Read the model definition and answer for the solid it produces. Units are mm, in the model's axes. Face numbers are marked on the shaded views. A direction names the side the tool comes from. Give positions to 0.01 mm unless a question says otherwise; leave off trailing zeros. Order: outer loops, then holes, each group sorted by start corner. A loop starts at its lowest first (then second) coordinate and runs counter-clockwise, first axis right, second up.
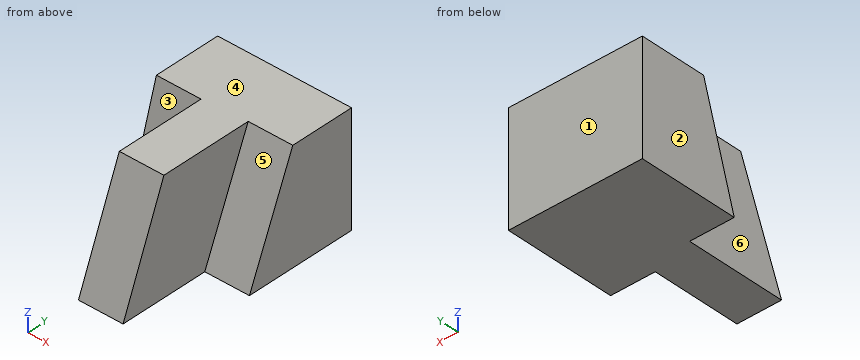
```python
from build123d import *

# Parameters (mm, degrees)
F0_W     = 38.1
F0_H     = 31.75
F1_DEPTH = 57.15
F3_DEPTH = 12.7
F5_DEPTH = 12.7
F7_DEPTH = 25.4


with BuildPart() as f1:
    # F0 (on Front) → F1 (new body)
    with BuildSketch(Plane.XZ):
        with Locations((19.05, 15.875)):
            Rectangle(F0_W, F0_H)
    extrude(amount=F1_DEPTH)

    # F2 (on face) → F3 (cut)
    with BuildSketch(Plane(origin=(0, 0, 0), x_dir=(0, -1, 0), z_dir=(-1, 0, 0))):
        Polygon((57.15, 31.75), (19.05, 31.75), (28.575, 0), (57.15, 0), align=None)
    extrude(amount=-F3_DEPTH, mode=Mode.SUBTRACT)

    # F4 (on face) → F5 (cut)
    with BuildSketch(Plane.YZ.offset(38.1)):
        Polygon((-31.75, 0), (-18.2607397437, 31.75), (-57.15, 31.75), (-57.15, 0), align=None)
    extrude(amount=-F5_DEPTH, mode=Mode.SUBTRACT)

    # F6 (on face) → F7 (cut)
    with BuildSketch(Plane(origin=(12.7, 0, 0), x_dir=(0, -1, 0), z_dir=(-1, 0, 0))):
        Polygon((57.15, 0), (57.15, 31.75), (44.45, 31.75), align=None)
    extrude(amount=-F7_DEPTH, mode=Mode.SUBTRACT)


solid = f1.part
```
1) The part is cut by section A-A on z = 19. Determine the outline of the cut face in (x, y) (3 decimals), and give its area (3 significant figures).
Final values:
outline: (0, -22.875) - (12.7, -22.875) - (12.7, -49.55) - (25.4, -49.55) - (25.4, -23.678) - (38.1, -23.678) - (38.1, 0) - (0, 0) - close
area: 1,220 mm2
2) The part is cut by section C-C on y = -36.5. Determine the outline of the cut face in (x, z), and give its area (3 significant figures).
Final values:
outline: (12.7, 0) - (25.4, 0) - (25.4, 31.75) - (12.7, 31.75) - close
area: 403 mm2
3) For a pull along Y with two mould halves and no side action, classify the marked faces 1, 2 and 3 as released by +Y, released by -Y, zero draft, split by the parting line, or undercut.
Final values:
face 1: released by +Y
face 2: zero draft
face 3: released by -Y
4) A tool of negligible diameter and unlimited length cuts with its end or side. For the marked faces 4, 5 and 6, from which of +Z, -Z, +X, -X, +Y, -Y can it reach the whole face along a straight path? Write none if from no direction.
Final values:
face 4: +Z, +X, -X, +Y, -Y
face 5: +Z, +X, -Y
face 6: +Z, -X, -Y
5) Given pin 1 (9.5 mm diameter, centred on y = -43, z = 14, fed in from +X); pin 2 (4 mm diameter, centred on x = 10.5, z = 6.5, fed in from -Y) (3 decimals); pin 3 (5 mm diameter, centred on x = 8, z = 15.5, fed in from -Y) (3 decimals), each flat-ended and moving along its own axis, determine where each tip first touches the part or whether it passes through.
Final values:
pin 1: stops at x = 25.4
pin 2: stops at y = -27.225
pin 3: stops at y = -24.675
6) The part is cut by section B-B on x = 17.5. Determine the outline of the cut face in (y, z).
Final values:
outline: (-57.15, 0) - (0, 0) - (0, 31.75) - (-44.45, 31.75) - close
7) The part is cut by section D-D on z = 12.5. Determine the outline of the cut face in (x, y) (3 decimals).
Final values:
outline: (0, -24.825) - (12.7, -24.825) - (12.7, -52.15) - (25.4, -52.15) - (25.4, -26.439) - (38.1, -26.439) - (38.1, 0) - (0, 0) - close
8) Consider L1, parallel to X at y = -41, z = 28.5; L2, parallel to Y at x = 2, z = 29 (3 decimals); L3, parallel to Y at x = 20, z = 29.5. Determine where each line is inside the solid, lowest interval first.
Final values:
L1: x = 12.7 to 25.4
L2: y = -19.875 to 0
L3: y = -45.35 to 0
